Work out the finished part from the listing and answer in its coordinate system (mm). Face numbers are marked on the shaded views. A direction names the side the tool comes from. Round coordinates to 2 decimals unless told otherwise and drop trailing zeros. Write each loop counter-clockwise with the first axis right and the second up, starting at its lowest first coordinate (ties: lowest second). Pieces come first, ordered by that corner, then holes. Notation, with made-up numbers: (-5, 82) -> (19, 82) arc R11 ccw to (19, 92) -> close; hole circle Ø1 at (30, 65.5). An arc over 180 degrees is marked (long way). One line per item, written item: value.
```python
from build123d import *

# Parameters (mm, degrees)
F0_W      = 25
F0_H      = 24
F0_R      = 1.1
F1_DEPTH  = 1
F2_R      = 0.92
F3_DEPTH  = 1
F2_W      = 8.4
F2_H      = 8.4
F2_R_2    = 3.75
F2_R_3    = 2.75
F4_DEPTH  = 1.65
F5_DEPTH  = 3.51
F6_DEPTH  = 4.51
F7_R      = 0.8
F8_DEPTH  = 0.1
F9_W      = 22
F9_H      = 6
F10_DEPTH = 2.65
F12_W     = 16
F12_H     = 3
F13_DEPTH = 0.1


with BuildPart() as f1:
    # F0 (on Top) → F1 (new body)
    with BuildSketch(Plane.XY):
        Rectangle(F0_W, F0_H)
        with Locations((-10.5, -3.5)):
            Circle(F0_R, mode=Mode.SUBTRACT)
        with Locations((10.5, -3.5)):
            Circle(F0_R, mode=Mode.SUBTRACT)
        with Locations((-10.5, 10)):
            Circle(F0_R, mode=Mode.SUBTRACT)
        with Locations((10.5, 10)):
            Circle(F0_R, mode=Mode.SUBTRACT)
    extrude(amount=F1_DEPTH)

    # F2 (on face) → F3 (cut, through all)
    with BuildSketch(Plane.XY.offset(1)):
        with Locations((-9, 3.25)):
            Circle(F2_R)
        with Locations((9, 3.25)):
            Circle(F2_R)
    extrude(amount=-F3_DEPTH, mode=Mode.SUBTRACT)

    # F2 (on face) → F4 (join)
    with BuildSketch(Plane.XY.offset(1)):
        with Locations((0, 3.25)):
            Rectangle(F2_W, F2_H)
        with Locations((0, 3.25)):
            Circle(F2_R_2, mode=Mode.SUBTRACT)
        with Locations((0, 3.25)):
            Circle(F2_R_2)
        with Locations((0, 3.25)):
            Circle(F2_R_3, mode=Mode.SUBTRACT)
        with Locations((0, 3.25)):
            Circle(F2_R_3)
    extrude(amount=F4_DEPTH)

    # F2 (on face) → F5 (join)
    with BuildSketch(Plane.XY.offset(1)):
        with Locations((0, 3.25)):
            Circle(F2_R_2)
        with Locations((0, 3.25)):
            Circle(F2_R_3, mode=Mode.SUBTRACT)
        with Locations((0, 3.25)):
            Circle(F2_R_3)
    extrude(amount=F5_DEPTH)

    # F2 (on face) → F6 (join)
    with BuildSketch(Plane.XY.offset(1)):
        with Locations((0, 3.25)):
            Circle(F2_R_3)
    extrude(amount=F6_DEPTH)

    # F7 (on face) → F8 (join)
    with BuildSketch(Plane.XY.offset(5.51)):
        with Locations((0, 3.25)):
            Circle(F7_R)
    extrude(amount=F8_DEPTH)

    # F9 (on face) → F10 (join)
    with BuildSketch(Plane.XY.offset(1)):
        with Locations((0, -9)):
            Rectangle(F9_W, F9_H)
    extrude(amount=F10_DEPTH)

    # F12 (on offset) → F13 (join)
    with BuildSketch(Plane(origin=(0, 0, 2.275), x_dir=(1, 0, 0), z_dir=(0, 0, -1))):
        with Locations((0, 13.5)):
            Rectangle(F12_W, F12_H)
    extrude(amount=F13_DEPTH)


solid = f1.part
```
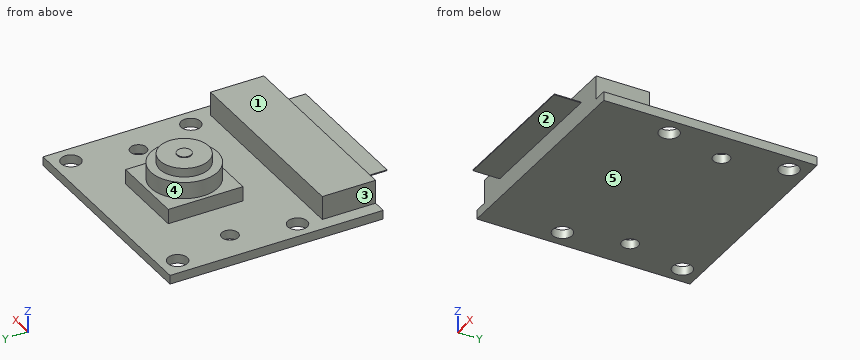
(1) Flat-ended cylindrical pins translate along their axes: pin 1 Ø3 at (x, y) = (10.5, -3.5) entering from +Z; pin 2 Ø0.5 at (y, z) = (5, 2) entering from -X; pin 3 Ø3 at (y, z) = (-11, 4) entering from +X. Find the tip coordinate at first contact, or state that the pin passes through.
Reported:
pin 1: stops at z = 1
pin 2: stops at x = -4.2
pin 3: stops at x = 11
(2) For a pull along Y with two mould halves and no side action, classify the marked faces 4 and 5 as pulls with the +Y half, pulls with the -Y half, needs draft (parallel to the pull), parting line crosses it, or undercut.
Reported:
face 4: undercut
face 5: needs draft
(3) Find section A-A on y = 3.25. Give the vertices of the cut face in (x, z).
Reported:
outline: (-12.5, 0) -> (-9.92, 0) -> (-9.92, 1) -> (-12.5, 1) -> close; (-8.08, 0) -> (8.08, 0) -> (8.08, 1) -> (4.2, 1) -> (4.2, 2.65) -> (3.75, 2.65) -> (3.75, 4.51) -> (2.75, 4.51) -> (2.75, 5.51) -> (0.8, 5.51) -> (0.8, 5.61) -> (-0.8, 5.61) -> (-0.8, 5.51) -> (-2.75, 5.51) -> (-2.75, 4.51) -> (-3.75, 4.51) -> (-3.75, 2.65) -> (-4.2, 2.65) -> (-4.2, 1) -> (-8.08, 1) -> close; (9.92, 0) -> (12.5, 0) -> (12.5, 1) -> (9.92, 1) -> close
(4) Find section D-D on y = -8.25. Give the vertices of the cut face in (x, z).
Reported:
outline: (-12.5, 0) -> (12.5, 0) -> (12.5, 1) -> (11, 1) -> (11, 3.65) -> (-11, 3.65) -> (-11, 1) -> (-12.5, 1) -> close
(5) Consider probe 1 along Y at (x, z) = (-10.5, 0.5); probe 2 along Y at (x, z) = (-3, 2.55); probe 3 along Z at (x, y) = (5.25, 0.5). Determine where each line is inside the solid, lowest interval first.
Reported:
probe 1: y = -12 to -4.6, -2.4 to 8.9, 11.1 to 12
probe 2: y = -12 to -6, -0.95 to 7.45
probe 3: z = 0 to 1
(6) A tool of negligible diameter and unlimited length cuts with its end or side. For the marked faces 1, 2 and 3, from which of +Z, -Z, +X, -X, +Y, -Y can it reach the whole face along a straight path? Write none if from no direction.
Reported:
face 1: +Z, +X, -X, -Y
face 2: -Z, +X, -X, -Y
face 3: +Z, -X, +Y, -Y
(7) Find section C-C on x = 9. Give the vertices of the cut face in (y, z).
Reported:
outline: (-12, 0) -> (2.33, 0) -> (2.33, 1) -> (-6, 1) -> (-6, 3.65) -> (-12, 3.65) -> close; (4.17, 0) -> (12, 0) -> (12, 1) -> (4.17, 1) -> close
(8) Find section B-B on z = 1.3. Give the vertices of the cut face in (x, y), plus the area to 3 significant figures.
Reported:
outline: (-11, -12) -> (11, -12) -> (11, -6) -> (-11, -6) -> close; (-4.2, -0.95) -> (4.2, -0.95) -> (4.2, 7.45) -> (-4.2, 7.45) -> close
area: 203 mm2
